from build123d import *

# Parameters (mm, degrees)
IZIM1_R                     = 15
Y_KSEKLIK_EKSTR_ZYON1_DEPTH = 25
IZIM2_R                     = 7.5
Y_KSEKLIK_EKSTR_ZYON2_DEPTH = 41
IZIM3_R                     = 5.5
Y_KSEKLIK_EKSTR_ZYON3_DEPTH = 4
IZIM4_R                     = 7.5
Y_KSEKLIK_EKSTR_ZYON4_DEPTH = 6
Y_KSEKLIK_EKSTR_ZYON5_START = 41
IZIM6_R                     = 7.5
Y_KSEKLIK_EKSTR_ZYON5_DEPTH = 41
Y_KSEKLIK_EKSTR_ZYON6_START = 4
IZIM7_R                     = 5.5
Y_KSEKLIK_EKSTR_ZYON6_DEPTH = 4
Y_KSEKLIK_EKSTR_ZYON7_START = 6
IZIM8_R                     = 7.5
Y_KSEKLIK_EKSTR_ZYON7_DEPTH = 6


with BuildPart() as part:
    # Çizim1 → Yükseklik-Ekstrüzyon1 (new, symmetric)
    with BuildSketch(Plane.XY):
        Circle(IZIM1_R)
    extrude(amount=Y_KSEKLIK_EKSTR_ZYON1_DEPTH, both=True)

    # Çizim2 → Yükseklik-Ekstrüzyon2 (add)
    with BuildSketch(Plane.XY.offset(25)):
        Circle(IZIM2_R)
    extrude(amount=Y_KSEKLIK_EKSTR_ZYON2_DEPTH)

    # Çizim3 → Yükseklik-Ekstrüzyon3 (add)
    with BuildSketch(Plane.XY.offset(66)):
        Circle(IZIM3_R)
    extrude(amount=Y_KSEKLIK_EKSTR_ZYON3_DEPTH)

    # Çizim4 → Yükseklik-Ekstrüzyon4 (add)
    with BuildSketch(Plane.XY.offset(70)):
        Circle(IZIM4_R)
    extrude(amount=Y_KSEKLIK_EKSTR_ZYON4_DEPTH)

    # Çizim6 → Yükseklik-Ekstrüzyon5 (add)
    with BuildSketch(Plane(origin=(0, 0, -25), x_dir=(-1, 0, 0), z_dir=(0, 0, -1)).offset(Y_KSEKLIK_EKSTR_ZYON5_START)):
        with Locations(Location((0, 0, 0), (0, 0, 180))):
            Circle(IZIM6_R)
    extrude(amount=-Y_KSEKLIK_EKSTR_ZYON5_DEPTH)

    # Çizim7 → Yükseklik-Ekstrüzyon6 (add)
    with BuildSketch(Plane(origin=(0, 0, -66), x_dir=(-1, 0, 0), z_dir=(0, 0, -1)).offset(Y_KSEKLIK_EKSTR_ZYON6_START)):
        with Locations(Location((0, 0, 0), (0, 0, 180))):
            Circle(IZIM7_R)
    extrude(amount=-Y_KSEKLIK_EKSTR_ZYON6_DEPTH)

    # Çizim8 → Yükseklik-Ekstrüzyon7 (add)
    with BuildSketch(Plane(origin=(0, 0, -70), x_dir=(-1, 0, 0), z_dir=(0, 0, -1)).offset(Y_KSEKLIK_EKSTR_ZYON7_START)):
        with Locations(Location((0, 0, 0), (0, 0, 180))):
            Circle(IZIM8_R)
    extrude(amount=-Y_KSEKLIK_EKSTR_ZYON7_DEPTH)


solid = part.part
Source: CAD feature listing. Evaluate the final solid. Frame: model axes, mm. A direction names the side the tool comes from. Coordinates: 2 decimals unless noted, no trailing zeros. Loops run counter-clockwise (first coordinate to the right, second up) from the corner with the lowest first, then second, coordinate; pieces in that order, holes last. Notation, with made-up numbers: (-2, 5) -> (38, 5) arc R7 ccw to (38, 14) -> close; hole circle Ø1 at (88.5, 36.5). An arc over 180 degrees is marked (long way). Answer in a Markdown table with one row per item. Add a question column.
Q1. Section D-D on y = 12. Return the cut outline in (x, z).
Q2. Pull-direction query (Z, two-part tool) for faces 1 (the face through (-1.19, -5.37, 67.97)), 2 (the face through (-7.493, 0.33, 72.958)), 3 (the face through (0, 0, 76)); classes: pulls with the +Z half, pulls with the -Z half, needs draft (parallel to the pull), parting line crosses it, or undercut.
Q3. Section C-C on z = 54. Return the cut outline in (x, y), and give its area (3 significant figures).
Q4. Contact query for flat-ended pins moving along their axis: pin 1 Ø10 at (y, z) = (7.5, -15) entering from -X; pin 2 Ø6 at (x, y) = (-3, -10.5) entering from -Z; pin 3 Ø1 at (x, z) = (-5, -29) entering from -Y. Output: stop coordinate, or through.
Q5. Reachability of faces 4 (the face through (-7.493, 0.33, 45.213)), 5 (the face through (-4, 4, 70)), 6 (the face through (-14.985, 0.66, 0.35)), 7 (the face through (4.032, -6.324, -45.787)) from +Z, -Z, +X, -X, +Y, -Y: full face, straight path, thin tool, end or side. Return the list, or none.
Q6. Section A-A on x = 0. Return the cut outline in (y, z), and give its area (3 significant figures).
Q7. Ray query, line 1 along Z through (x, y) = (-4, 5); line 2 along X through (y, z) = (0.5, 38.5); line 3 along X through (y, z) = (-0.75, 7.5). Return the intervals inside material, ascending.
Computed values:
| question | item | result |
|---|---|---|
| 1 | outline | (-9, -25) -> (9, -25) -> (9, 25) -> (-9, 25) -> close |
| 2 | face 1 | undercut |
| 2 | face 2 | needs draft |
| 2 | face 3 | pulls with the +Z half |
| 3 | outline | circle Ø15 at (0, 0) |
| 3 | area | 177 mm^2 |
| 4 | pin 1 | stops at x = -14.79 |
| 4 | pin 2 | stops at z = -25 |
| 4 | pin 3 | stops at y = -6 |
| 5 | face 4 | +Z |
| 5 | face 5 | none |
| 5 | face 6 | +Z, -Z |
| 5 | face 7 | -Z |
| 6 | outline | (-15, -25) -> (-7.5, -25) -> (-7.5, -66) -> (-5.5, -66) -> (-5.5, -70) -> (-7.5, -70) -> (-7.5, -76) -> (7.5, -76) -> (7.5, -70) -> (5.5, -70) -> (5.5, -66) -> (7.5, -66) -> (7.5, -25) -> (15, -25) -> (15, 25) -> (7.5, 25) -> (7.5, 66) -> (5.5, 66) -> (5.5, 70) -> (7.5, 70) -> (7.5, 76) -> (-7.5, 76) -> (-7.5, 70) -> (-5.5, 70) -> (-5.5, 66) -> (-7.5, 66) -> (-7.5, 25) -> (-15, 25) -> close |
| 6 | area | 3,000 mm^2 |
| 7 | line 1 | z = -76 to -70, -66 to 66, 70 to 76 |
| 7 | line 2 | x = -7.48 to 7.48 |
| 7 | line 3 | x = -14.98 to 14.98 |
